from build123d import *

# Parameters (mm, degrees)
F0_W     = 50.8
F0_H     = 152.4
F0_R     = 3.175
F0_R_2   = 2.032
F0_R_3   = 13.97
F1_DEPTH = 5.334
F2_R     = 3.175
F3_DEPTH = 25.4


with BuildPart() as f1:
    # F0 (on Top) → F1 (new body)
    with BuildSketch(Plane.XY):
        with Locations((-18.054181, 9.979866)):
            Rectangle(F0_W, F0_H)
        with Locations((-30.754181, -48.440134)):
            Circle(F0_R, mode=Mode.SUBTRACT)
        with Locations((-5.354181, -48.440134)):
            Circle(F0_R, mode=Mode.SUBTRACT)
        with Locations((-18.377712, 42.822066)):
            Circle(F0_R_2, mode=Mode.SUBTRACT)
        with Locations((-36.011981, 61.103397)):
            Circle(F0_R_2, mode=Mode.SUBTRACT)
        with Locations((-18.054181, 60.779866)):
            Circle(F0_R_3, mode=Mode.SUBTRACT)
        with Locations((-17.730651, 78.737666)):
            Circle(F0_R_2, mode=Mode.SUBTRACT)
        with Locations((-0.096381, 60.456336)):
            Circle(F0_R_2, mode=Mode.SUBTRACT)
    extrude(amount=F1_DEPTH)

    # F2 (on face) → F3 (cut)
    with BuildSketch(Plane(origin=(0, 0, 0), x_dir=(1, 0, 0), z_dir=(0, 0, -1))):
        with Locations((-5.354181, 48.440134)):
            Circle(F2_R)
        with Locations((-30.754181, 48.440134)):
            Circle(F2_R)
    extrude(amount=-F3_DEPTH, mode=Mode.SUBTRACT)


solid = f1.part
Geometry: final body of the model. Coordinates: model frame, mm. Give positions to 0.01 mm unless a question says otherwise; leave off trailing zeros. Write each loop counter-clockwise with the first axis right and the second up, starting at its lowest first coordinate (ties: lowest second). Pieces come first, ordered by that corner, then holes. Notation, with made-up numbers: M 21.5,-15.75 L 66.5,-15.75 A8 ccw 66.5,-5.75 Z; hole C 28.5,68 d10. An arc over 180 degrees is marked long. Answer in a Markdown table with one row per item. Add a question column.
(1) Ray query, line 1 (Y direction, x = -36, z = 3.85); line 2 (Y direction, x = -28, z = 3); line 3 (Y direction, x = -6, z = 0.85). Return the intervals inside material, ascending.
(2) Section A-A on x = -25. Return loops of the section in (y, z).
(3) Mould query, pull axis Y, two halves, no side actions, for faces 1 (the flat face through (-18, 86.18, 3)), 2 (the flat face through (-43.454, 9, 3)), 3 (the cylindrical face through (-0.36, 62.47, 2.63)), 4 (the flat face through (-18, -66.22, 3)). Classes: +Y half, -Y half, draft (parallel to the pull), parting line (faces both ways), or undercut.
(4) First-contact query: pin 1 (1.5 mm diameter, centred on x = -25, y = 19.5, fed in from -Z). Flat tip, straight axial feed; report the tip coordinate or a pass-through.
(5) Section B-B on z = 1.55. Return loops of the section in (x, y) (3 decimals).
(6) Section C-C on x = -13.5. Return loops of the section in (y, z).
Result set:
| question | item | result |
|---|---|---|
| 1 | line 1 | y = -66.22 to 59.07, 63.14 to 86.18 |
| 1 | line 2 | y = -66.22 to -50.02, -46.86 to 50.97, 70.59 to 86.18 |
| 1 | line 3 | y = -66.22 to -51.55, -45.33 to 53.72, 67.84 to 86.18 |
| 2 | outline | M -66.22,0 L 48.66,0 L 48.66,5.33 L -66.22,5.33 Z; M 72.9,0 L 86.18,0 L 86.18,5.33 L 72.9,5.33 Z |
| 3 | face 1 | +Y half |
| 3 | face 2 | draft |
| 3 | face 3 | undercut |
| 3 | face 4 | -Y half |
| 4 | pin 1 | stops at z = 0 |
| 5 | outline | M -43.454,-66.22 L 7.346,-66.22 L 7.346,86.18 L -43.454,86.18 Z; hole C -36.012,61.103 d4.064; hole C -30.754,-48.44 d6.35; hole C -18.054,60.78 d27.94; hole C -18.378,42.822 d4.064; hole C -17.731,78.738 d4.064; hole C -5.354,-48.44 d6.35; hole C -0.096,60.456 d4.064 |
| 6 | outline | M -66.22,0 L 47.57,0 L 47.57,5.33 L -66.22,5.33 Z; M 73.99,0 L 86.18,0 L 86.18,5.33 L 73.99,5.33 Z |
